Model file for the job. Use its own axes, mm. A direction names the side the tool comes from. Give positions to 0.01 mm unless a question says otherwise; leave off trailing zeros. Loops run counter-clockwise (first coordinate to the right, second up) from the corner with the lowest first, then second, coordinate; pieces in that order, holes last. Notation, with made-up numbers: M 87,27 L 134,27 A32 cw 134,53 Z; hole C -17.5,79 d1. An arc over 180 degrees is marked long. Answer in a Markdown table with one row per item.
```python
from build123d import *

# Parameters (mm, degrees)
SKETCH1_W           = 73.2
SKETCH1_H           = 73.2
SKETCH1_W_2         = 70.2
SKETCH1_H_2         = 70.2
BOSS_EXTRUDE1_DEPTH = 5
SKETCH2_W           = 73.2
SKETCH2_H           = 73.2
BOSS_EXTRUDE2_DEPTH = 1.6
FILLET1_R           = 6.6
SKETCH3_W           = 50
SKETCH3_H           = 50
CUT_EXTRUDE1_DEPTH  = 1.6
FILLET2_R           = 6.6
SKETCH5_W           = 35
SKETCH5_H           = 12.4
BOSS_EXTRUDE3_DEPTH = 7
SKETCH6_W           = 24
SKETCH6_H           = 12.4
CUT_EXTRUDE2_DEPTH  = 1.8
SKETCH7_W           = 17
SKETCH7_H           = 12.4
CUT_EXTRUDE3_DEPTH  = 10.8
SKETCH8_W           = 35
SKETCH8_H           = 7
BOSS_EXTRUDE4_DEPTH = 1
FILLET3_R           = 8.1
FILLET4_R           = 3
FILLET5_R           = 6
SKETCH9_R           = 0.7
CUT_EXTRUDE4_DEPTH  = 10


with BuildPart() as part:
    # Sketch1 → Boss-Extrude1 (new body)
    with BuildSketch(Plane.XY):
        with Locations((35.1, 35.1)):
            Rectangle(SKETCH1_W, SKETCH1_H)
        with Locations((35.1, 35.1)):
            Rectangle(SKETCH1_W_2, SKETCH1_H_2, mode=Mode.SUBTRACT)
    extrude(amount=BOSS_EXTRUDE1_DEPTH)

    # Sketch2 → Boss-Extrude2 (add)
    with BuildSketch(Plane.XY.offset(5)):
        with Locations((35.1, 35.1)):
            Rectangle(SKETCH2_W, SKETCH2_H)
    extrude(amount=BOSS_EXTRUDE2_DEPTH)

    # Fillet1
    fillet1_edges = [part.edges().sort_by_distance(p)[0] for p in [
        (0, 70.2, 2.5),
        (0, 0, 2.5),
        (70.2, 0, 2.5),
        (70.2, 70.2, 2.5),
    ]]
    fillet(fillet1_edges, radius=FILLET1_R)

    # Sketch3 → Cut-Extrude1 (cut)
    with BuildSketch(Plane(origin=(0, 0, 5), x_dir=(-1, 0, 0), z_dir=(0, 0, -1))):
        with Locations((-42.2, 28)):
            Rectangle(SKETCH3_W, SKETCH3_H)
    extrude(amount=-CUT_EXTRUDE1_DEPTH, mode=Mode.SUBTRACT)

    # Fillet2
    fillet2_edges = [part.edges().sort_by_distance(p)[0] for p in [
        (67.2, 3, 5.8),
        (67.2, 53, 5.8),
        (17.2, 53, 5.8),
        (17.2, 3, 5.8),
    ]]
    fillet(fillet2_edges, radius=FILLET2_R)

    # Sketch5 → Boss-Extrude3 (add)
    with BuildSketch(Plane.XY.offset(6.6)):
        with Locations((54.2, 77.9)):
            Rectangle(SKETCH5_W, SKETCH5_H)
    extrude(amount=-BOSS_EXTRUDE3_DEPTH)

    # Sketch6 → Cut-Extrude2 (cut)
    with BuildSketch(Plane(origin=(0, 0, -0.4), x_dir=(-1, 0, 0), z_dir=(0, 0, -1))):
        with Locations((-54.2, 77.9)):
            Rectangle(SKETCH6_W, SKETCH6_H)
    extrude(amount=-CUT_EXTRUDE2_DEPTH, mode=Mode.SUBTRACT)

    # Sketch7 → Cut-Extrude3 (cut)
    with BuildSketch(Plane(origin=(0, 0, 1.4), x_dir=(-1, 0, 0), z_dir=(0, 0, -1))):
        with Locations((-57.7, 77.9)):
            Rectangle(SKETCH7_W, SKETCH7_H)
    extrude(amount=-CUT_EXTRUDE3_DEPTH, mode=Mode.SUBTRACT)

    # Sketch8 → Boss-Extrude4 (add)
    with BuildSketch(Plane(origin=(0, 84.1, 0), x_dir=(1, 0, 0), z_dir=(0, 1, 0))):
        with Locations((54.2, -3.1)):
            Rectangle(SKETCH8_W, SKETCH8_H)
    extrude(amount=BOSS_EXTRUDE4_DEPTH)

    # Fillet3
    fillet3_edges = [part.edges().sort_by_distance(p)[0] for p in [
        (71.7, -1.5, 3.3),
        (-1.5, -1.5, 3.3),
        (-1.5, 71.7, 3.3),
    ]]
    fillet(fillet3_edges, radius=FILLET3_R)

    # Fillet4
    fillet4_edges = [part.edges().sort_by_distance(p)[0] for p in [
        (71.7, 85.1, 3.1),
        (36.7, 85.1, 3.1),
        (36.7, 71.7, 3.3),
    ]]
    fillet(fillet4_edges, radius=FILLET4_R)

    # Fillet5
    fillet5_edges = [part.edges().sort_by_distance(p)[0] for p in [
        (49.2, 84.1, 4),
        (49.2, 71.7, 4),
    ]]
    fillet(fillet5_edges, radius=FILLET5_R)

    # Sketch9 → Cut-Extrude4 (cut)
    with BuildSketch(Plane(origin=(0, 0, -0.4), x_dir=(-1, 0, 0), z_dir=(0, 0, -1))):
        with Locations((-40.448812376, 78.1)):
            Circle(SKETCH9_R)
        with Locations((-67.948812376, 78.1)):
            Circle(SKETCH9_R)
    extrude(amount=-CUT_EXTRUDE4_DEPTH, mode=Mode.SUBTRACT)


solid = part.part
```
Q1. Saw through at C-C (y = 61). Give the cut face in (x, z), and give its area (3 significant figures).
Reported:
| item | result |
|---|---|
| outline | M -1.5,0 L 0,0 L 0,5 L 70.2,5 L 70.2,0 L 71.7,0 L 71.7,6.6 L -1.5,6.6 Z |
| area | 132 mm² |
Q2. Drop flat-ended pins along their axis: pin 1 (2 mm diameter, centred on x = 7.5, z = 0.5, fed in from +Y); pin 2 (3.5 mm diameter, centred on x = 46.5, y = 76.5, fed in from -Z); pin 3 (3 mm diameter, centred on x = 8.5, y = 45.5, fed in from -Z). Give the stop position or say it passes through.
Reported:
| item | result |
|---|---|
| pin 1 | y = 71.7 |
| pin 2 | z = 1.4 |
| pin 3 | z = 5 |
Q3. Saw through at A-A (z = 4). Give the cut face in (x, y), and give its area (3 significant figures).
Reported:
| item | result |
|---|---|
| outline | M -1.5,6.6 A8.1 ccw 6.6,-1.5 L 63.6,-1.5 A8.1 ccw 71.7,6.6 L 71.7,82.1 A3 ccw 68.7,85.1 L 39.7,85.1 A3 ccw 36.7,82.1 L 36.7,74.7 A3 cw 33.7,71.7 L 6.6,71.7 A8.1 ccw -1.5,63.6 Z; hole M 0,6.6 A6.6 ccw 6.6,0 L 63.6,0 A6.6 ccw 70.2,6.6 L 70.2,63.6 A6.6 ccw 63.6,70.2 L 6.6,70.2 A6.6 ccw 0,63.6 Z; hole C 40.45,78.1 d1.4; hole M 49.2,77.7 A6 ccw 55.2,71.7 L 66.2,71.7 L 66.2,84.1 L 55.2,84.1 A6 ccw 49.2,78.1 Z; hole C 67.95,78.1 d1.4 |
| area | 694 mm² |
Q4. Probe probe 1 along X at (y, z) = (78.1, 2.75); probe 2 along Y at (x, z) = (63, 4.5); probe 3 along X at (y, z) = (14.5, 2). List the from-to ranges inside material, lowest first.
Reported:
| item | result |
|---|---|
| probe 1 | 36.7 to 39.75, 41.15 to 49.2, 66.2 to 67.25, 68.65 to 71.7 |
| probe 2 | -1.5 to 0, 70.2 to 71.7, 84.1 to 85.1 |
| probe 3 | -1.5 to 0, 70.2 to 71.7 |
Q5. 3-axis set-ups, long thin cutter, end or side, ignore diameter. For faces 1 (the face through (19, 51.2, 5)), 2 (the face through (65.318, 4.985, 5.811)), 3 (the face through (20, 71.7, 3)): which of +Z, -Z, +X, -X, +Y, -Y reach the whole face in a straight line?
Reported:
| item | result |
|---|---|
| face 1 | -Z |
| face 2 | +Z, -Z |
| face 3 | +Z, -Z, -X, +Y |
Q6. Saw through at B-B (y = 42). Give the cut face in (x, z), and give its area (3 significant figures).
Reported:
| item | result |
|---|---|
| outline | M -1.5,0 L 0,0 L 0,5 L 17.2,5 L 17.2,6.6 L -1.5,6.6 Z; M 67.2,5 L 70.2,5 L 70.2,0 L 71.7,0 L 71.7,6.6 L 67.2,6.6 Z |
| area | 52.1 mm² |
Q7. Mould opens along Y. For faces 4 (the face through (46, 78, 1.4)), 5 (the face through (24, 71, 0)), 6 (the face through (37.6, 84.24, 3.05)), 7 (the face through (50.911, 73.504, 4.036)) say: released by +Y, released by -Y, zero draft, split by the parting line, or undercut.
Reported:
| item | result |
|---|---|
| face 4 | undercut |
| face 5 | zero draft |
| face 6 | released by +Y |
| face 7 | undercut |
Q8. Saw through at D-D (x = 3). Give the cut face in (y, z), and give its area (3 significant figures).
Reported:
| item | result |
|---|---|
| outline | M -0.66,0 L 1.07,0 L 1.07,5 L 69.13,5 L 69.13,0 L 70.86,0 L 70.86,6.6 L -0.66,6.6 Z |
| area | 132 mm² |
